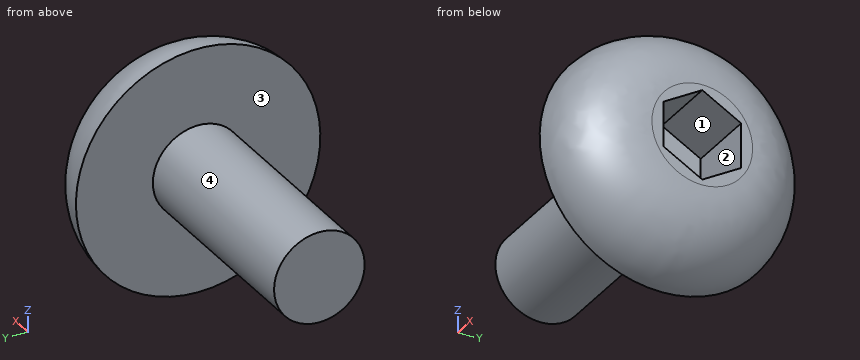
Autodesk Inventor part; units mm, degrees
ref_plane "YZ Plane" through (0, 0, 0) normal (1, 0, 0) x (0, 1, 0)
ref_plane "XZ Plane" through (0, 0, 0) normal (0, 1, 0) x (-1, 0, 0)
ref_plane "XY Plane" through (0, 0, 0) normal (0, 0, 1) x (1, 0, 0)
sketch "Sketch1" plane through (0, 0, 0) normal (1, 0, 0) x (0, 1, 0)
  circle A0 centre (0, 0) radius 2
  dimension "d0" = 4
extrude "Extrusion1" add sketch "Sketch1" along normal blind 9.525
sketch "Sketch2" plane through (9.525, 0, 0) normal (1, 0, 0) x (0, 0, -1)
  circle A0 centre (0, 0) radius 5.3975
  dimension "d3" = 10.795
extrude "Extrusion2" add sketch "Sketch2" along normal blind 3.175
sketch "Sketch3" plane through (12.7, 0, 0) normal (1, 0, 0) x (0, 0, -1)
  line L0 (0, 0) -> (1.9812, 0)
  line L1 (0, 0) -> (-1.9812, 0)
  circle A0 centre (0, 0) radius 2
  line L2 (0, 0) -> (0.9906, 1.7158)
  line L3 (0, 0) -> (1.9812, 0) construction
  line L4 (0.9906, 1.7158) -> (1.9812, 0)
  line L5 (0, 0) -> (-0.9906, 1.7158)
  line L6 (0, 0) -> (1.9812, 0) construction
  line L7 (-0.9906, 1.7158) -> (0.9906, 1.7158)
  line L8 (-0.9906, 1.7158) -> (-1.9812, 0)
  line L9 (0, 0) -> (0.9906, -1.7158)
  line L10 (0, 0) -> (1.9812, 0) construction
  line L11 (0.9906, -1.7158) -> (1.9812, 0)
  line L12 (0, 0) -> (-0.9906, -1.7158)
  line L13 (0, 0) -> (1.9812, 0) construction
  line L14 (-0.9906, -1.7158) -> (0.9906, -1.7158)
  line L15 (-0.9906, -1.7158) -> (-1.9812, 0)
  dimension "d6" = 1.9812
  dimension "d7" = 1.9812
  dimension "d8" = 1.9812
  dimension "d9" = 60
  dimension "d10" = 1.9812
  dimension "d11" = 120
  dimension "d12" = 1.9812
  dimension "d13" = 60
  dimension "d14" = 1.9812
  dimension "d15" = 120
extrude "Extrusion3" cut sketch "Sketch3" against normal blind 3.175 contours L2 L4 L0 | L12 L15 L1 | L5 L7 L2 | L1 L8 L5 | L0 L11 L9 | L9 L14 L12
fillet "Fillet1" radius 3.175 1 edges at (12.7, 0, 5.3975)
thread "Thread1"
properties part number "4M Screw"
Part model, mm, in its own coordinate system. Face numbers are marked on the shaded views. Give positions to 0.01 mm unless a question says otherwise; leave off trailing zeros. Loops run counter-clockwise (first coordinate to the right, second up) from the corner with the lowest first, then second, coordinate; pieces in that order, holes last. Notation, with made-up numbers: (75, 65) -> (112, 65) arc R30 ccw to (112, 96) -> close; hole circle Ø4 at (73.25, -15). An arc over 180 degrees is marked (long way). Write each question's results on one line, items separated by ' | '. Start each with the question number.
Q1. Wall check: L1, parallel to X at y = 1, z = 2 (3 decimals); L2, parallel to X at y = -0.25, z = -1 (3 decimals); L3, parallel to Y at x = 10.75, z = -1.75. Give the ranges that are in metal, low to high.
Q2. Band-saw the part on A-A on x = 3.5. List the corners of the cut face in (y, z), plus the area to 3 significant figures.
Q3. Pull direction Z, two halves, no side cores. Call the marked faces 1, 2, 3 and 4: +Z half, -Z half, draft (parallel to the pull), parting line (faces both ways), or undercut.
Q4. Pin check, flat tips, straight feed: P1, Ø1, axis at x = 4.5, y = 3, coming from the +Z side; P2, Ø4, axis at x = 9, y = 4, coming from the +Z side; P3, Ø2.5, axis at y = 0, z = 0, coming from the +X side (3 decimals); P4, Ø1.6, axis at x = 11.5, z = 0, coming from the +Y side. Stop position of each tip, or through.
Results are:
1) L1: x = 9.525 to 12.7 | L2: x = 0 to 9.525 | L3: y = -4.85 to -0.4, 0.4 to 4.85
2) outline: circle Ø4 at (0, 0) | area: 12.6 mm²
3) face 1: undercut | face 2: undercut | face 3: draft | face 4: parting line
4) P1: passes through | P2: stops at z = 4.98 | P3: stops at x = 9.525 | P4: stops at y = 5.17
